Check sheet for the drawn part. Datum: minimum x, y, z corner. Units: mm. Round coordinates to 2 decimals unless told otherwise and drop trailing zeros. Order: outer loops, then holes, each group sorted by start corner. A loop starts at its lowest first (then second) coordinate and runs counter-clockwise, first axis right, second up. Notation, with made-up numbers: (3.25, 44) -> (24.25, 44) arc R8 cw to (24.25, 59) -> close; hole circle Ø9 at (74, 56). An arc over 180 degrees is marked (long way). Answer in a Markdown table with one row per item.
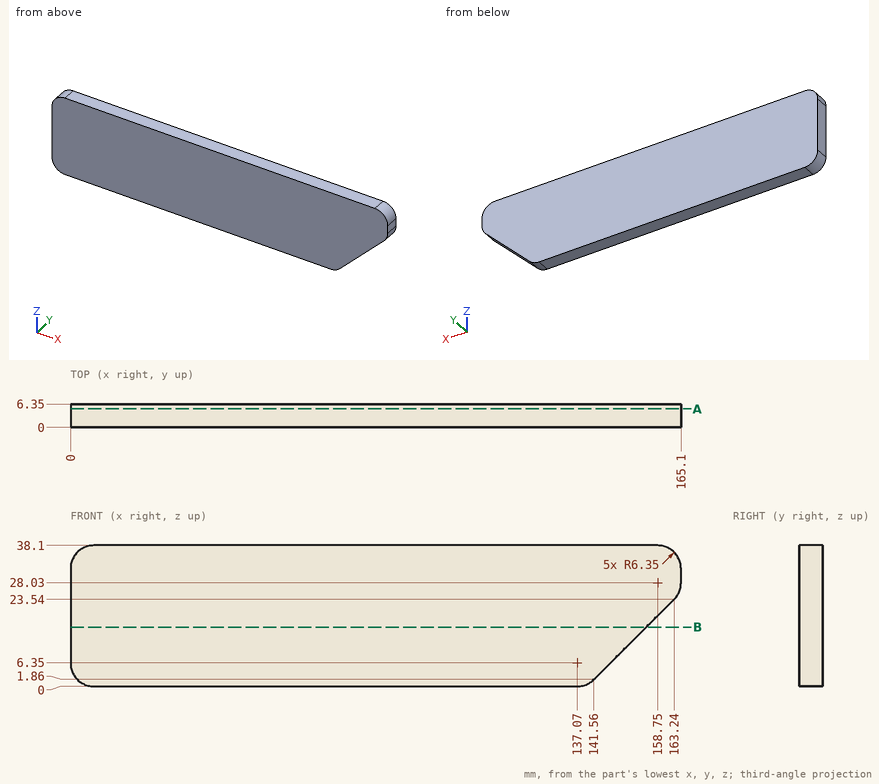
(1) Scan lines: probe 1 along X at (y, z) = (2.5, 9); probe 2 along X at (y, z) = (3.75, 6). Record each from-to range of solid material in increasing order. Write a range as from..to.
Solutions:
| item | result |
|---|---|
| probe 1 | 0..148.7 |
| probe 2 | 0.01..145.7 |
(2) Section check B-B on z = 16. Record the boundary of the cut face in (x, y), plus the area to 3 significant figures.
Solutions:
| item | result |
|---|---|
| outline | (0, 0) -> (155.7, 0) -> (155.7, 6.35) -> (0, 6.35) -> close |
| area | 989 mm^2 |
(3) Section check A-A on y = 5. Record the boundary of the cut face in (x, z), plus the area to 3 significant figures.
Solutions:
| item | result |
|---|---|
| outline | (0, 6.35) arc R6.35 ccw to (6.35, 0) -> (137.07, 0) arc R6.35 ccw to (141.56, 1.86) -> (163.24, 23.54) arc R6.35 ccw to (165.1, 28.03) -> (165.1, 31.75) arc R6.35 ccw to (158.75, 38.1) -> (6.35, 38.1) arc R6.35 ccw to (0, 31.75) -> close |
| area | 5,940 mm^2 |
